Check sheet for the modelled part. Datum: model origin and axes. Units: mm. A direction names the side the tool comes from. Coordinates: 2 decimals unless noted, no trailing zeros. Loops run counter-clockwise (first coordinate to the right, second up) from the corner with the lowest first, then second, coordinate; pieces in that order, holes last. Notation, with made-up numbers: (-20.75, 3) -> (8.25, 3) arc R20 cw to (8.25, 36) -> close; hole circle Ø8 at (23.25, -4). An arc over 180 degrees is marked (long way). Use CSV: the item, a comma, the result in double quotes. Start each with the question number.
1. Sectioned sample at A-A, the plane x = 10. Record the cut outline in (y, z).
2. Sectioned sample at D-D, the plane x = 421. Record the cut outline in (y, z).
3. Sectioned sample at C-C, the plane z = 10. Record the cut outline in (x, y), and give its area (3 significant figures).
4. Release check for a two-part mould opening along X. For faces 4 (the face through (243.7, 9.9, 169.2)), 5 (the face through (471, 10, 210)), 6 (the face through (13.55, 10.37, 53.87)) record: pulls with the +X half, pulls with the -X half, needs draft (parallel to the pull), parting line crosses it, or undercut.
5. Set-up check for faces 1 (the face through (90, 10, 80)), 2 (the face through (420, 90, 161)), 3 (the face through (411.46, 54.65, 208)): record each of +Z, -Z, +X, -X, +Y, -Y from which the full face is reachable in a straight line by a thin tool's end or side.
6. Gauge pin test, flat ends, axial feed: pin 1 (22 mm diameter, centred on y = 92, z = 231.5, fed in from +X); pin 2 (22 mm diameter, centred on y = 88, z = 66.5, fed in from -X); pin 3 (6 mm diameter, centred on x = 43, y = 9.5, fed in from +Z); pin 4 (22 mm diameter, centred on x = 435.5, y = 87, fed in from -Z). Record the tip position at first contact, or that the pin passes through.
7. Thickness scan on L1, parallel to Y at x = 420.5, z = 198; L2, parallel to Z at x = 50, y = 10.25; L3, parallel to Z at x = 10, y = 12.5. Record the ranges inside material, lowest first.
8. Sectioned sample at B-B, the plane y = 10.5. Record the cut outline in (x, z), and give its area (3 significant figures).
Solid Edge part; units mm, degrees
sketch "Sketch1" plane through (0, 0, 0) normal (0, -1, 0) x (1, 0, 0)
  line L0 (471, 261) -> (371, 261)
  line L1 (120, 80) -> (371, 261)
  line L2 (60, 80) -> (120, 80)
  line L3 (60, 60) -> (60, 80)
  line L4 (0, 60) -> (60, 60)
  line L5 (0, 0) -> (0, 60)
  line L6 (0, 0) -> (60, 0)
  line L7 (60, 0) -> (60, -20)
  line L8 (60, -20) -> (120, -20)
  line L9 (120, -20) -> (371, 161)
  line L10 (371, 161) -> (471, 161)
  line L11 (471, 161) -> (471, 261)
extrude "Protrusion1" add sketch "Sketch1" against normal blind 20
sketch "Sketch2" plane through (371, 20, 161) normal (0, -1, 0) x (1, 0, 0)
  circle A0 centre (50, 50) radius 10
extrude "Extrusionsausprägung_2" add sketch "Sketch2" against normal blind 7
sketch "Sketch3" plane through (421, 27, 211) normal (0, 1, 0) x (-1, 0, 0)
  circle A0 centre (0, 0) radius 100
extrude "Extrusionsausprägung_4" add sketch "Sketch3" along normal blind 3
sketch "Sketch4" plane through (421, 30, 211) normal (0, 1, 0) x (-1, 0, 0)
  circle A0 centre (0, 0) radius 10
extrude "Extrusionsausprägung_5" add sketch "Sketch4" along normal blind 50
sketch "Sketch5" plane through (421, 80, 211) normal (0, 1, 0) x (-1, 0, 0)
  line L0 (50, 50) -> (301, -131)
  line L1 (301, -131) -> (361, -131)
  line L2 (361, -131) -> (361, -151)
  line L3 (361, -151) -> (421, -151)
  line L4 (421, -151) -> (421, -211)
  line L5 (421, -211) -> (361, -211)
  line L6 (361, -211) -> (361, -231)
  line L7 (361, -231) -> (301, -231)
  line L8 (301, -231) -> (50, -50)
  line L9 (50, -50) -> (-50, -50)
  line L10 (-50, -50) -> (-50, 50)
  line L11 (-50, 50) -> (50, 50)
extrude "Extrusionsausprägung_6" add sketch "Sketch5" along normal blind 20
hole "Bohrung_1" at (10, 0, 50) direction (0, 1, 0) diameter 10.5 end up to next start chamfer 1 start chamfer angle 45
hole "Hole1" at (50, 0, 10) direction (0, 1, 0) diameter 10.5 end up to next start chamfer 1 start chamfer angle 45
hole "Bohrung_3" at (50, 100, 50) direction (0, -1, 0) diameter 10.5 end up to next start chamfer 1 start chamfer angle 45
hole "Hole2" at (10, 100, 10) direction (0, -1, 0) diameter 10.5 end up to next start chamfer 1 start chamfer angle 45
Completed:
1,outline,"(0, 0) -> (20, 0) -> (20, 44.75) -> (1, 44.75) -> (0, 43.75) -> close; (0, 56.25) -> (1, 55.25) -> (20, 55.25) -> (20, 60) -> (0, 60) -> close; (80, 0) -> (100, 0) -> (100, 3.75) -> (99, 4.75) -> (80, 4.75) -> close; (80, 15.25) -> (99, 15.25) -> (100, 16.25) -> (100, 60) -> (80, 60) -> close"
2,outline,"(0, 161) -> (20, 161) -> (20, 201) -> (27, 201) -> (27, 111) -> (30, 111) -> (30, 201) -> (80, 201) -> (80, 161) -> (100, 161) -> (100, 261) -> (80, 261) -> (80, 221) -> (30, 221) -> (30, 311) -> (27, 311) -> (27, 221) -> (20, 221) -> (20, 261) -> (0, 261) -> close"
3,outline,"(0, 0) -> (43.75, 0) -> (44.75, 1) -> (44.75, 20) -> (0, 20) -> close; (0, 80) -> (4.75, 80) -> (4.75, 99) -> (3.75, 100) -> (0, 100) -> close; (15.25, 80) -> (161.6, 80) -> (161.6, 100) -> (16.25, 100) -> (15.25, 99) -> close; (55.25, 1) -> (56.25, 0) -> (161.6, 0) -> (161.6, 20) -> (55.25, 20) -> close"
3,area,"6,040 mm²"
4,face 4,"pulls with the -X half"
4,face 5,"pulls with the +X half"
4,face 6,"undercut"
5,face 1,"+Z, -X, +Y, -Y"
5,face 2,"-Z, +X, +Y"
5,face 3,"none"
6,pin 1,"x = 471"
6,pin 2,"x = 0"
6,pin 3,"z = 60"
6,pin 4,"z = 161"
7,L1,"0 to 20, 27 to 30, 80 to 100"
7,L2,"0 to 4.75, 15.25 to 60"
7,L3,"0 to 44.75, 55.25 to 60"
8,outline,"(0, 0) -> (60, 0) -> (60, -20) -> (120, -20) -> (371, 161) -> (471, 161) -> (471, 261) -> (371, 261) -> (120, 80) -> (60, 80) -> (60, 60) -> (0, 60) -> close; hole circle Ø10.5 at (10, 50); hole circle Ø10.5 at (50, 10)"
8,area,"44,500 mm²"
